Print and shaded views of the part. All mm, measured from the part's lowest x, y and z. Coordinates: 2 decimals unless noted, no trailing zeros. Loops run counter-clockwise (first coordinate to the right, second up) from the corner with the lowest first, then second, coordinate; pieces in that order, holes last. Notation, with made-up numbers: M 88.5,-6.5 L 111.5,-6.5 A24 cw 111.5,20.5 Z; hole C 87.25,-2.5 d8. An arc over 180 degrees is marked long. Use a Markdown table: item, result. Add a question column.
1) Pin check, flat tip, straight feed: pin 1 Ø1.1 at (x, z) = (1, 6.08) entering from -Y (3 decimals). Stop position of the tip, or through.
2) Band-saw the part on C-C (y = 0.7). State how many separate pieces and enclosed holes the cut face has, plus the area to 3 significant figures.
3) Band-saw the part on B-B (z = 8.62). List the corners of the cut face in (x, y) (3 decimals), plus the area to 3 significant figures.
4) Band-saw the part on D-D (x = 6). List the corners of the cut face in (y, z).
5) Wall check: probe 1 along Z at (x, y) = (1, 0.8) (3 decimals); probe 2 along Z at (x, y) = (5.75, 0.1). Give the ranges that are in metal, low to high. Write a range as from..to.
6) Band-saw the part on A-A (x = 13.7). List the corners of the cut face in (y, z) (3 decimals), plus the area to 3 significant figures.
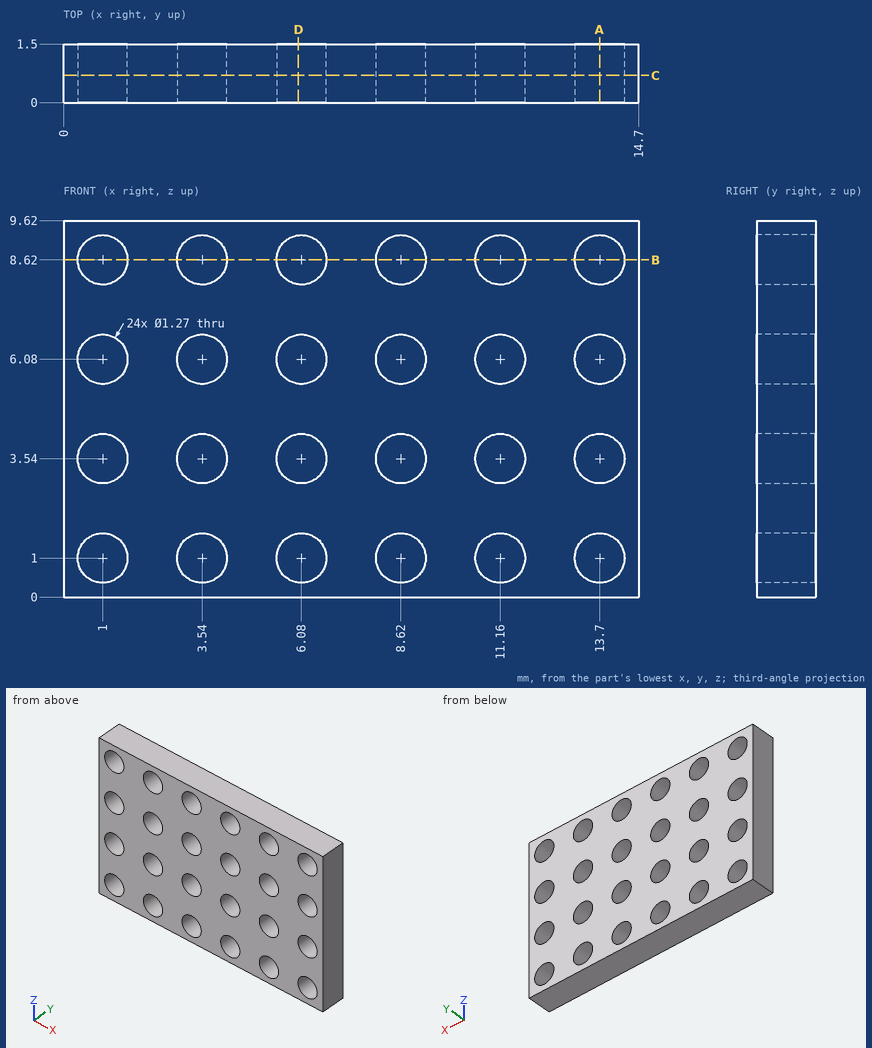
Entries:
| question | item | result |
|---|---|---|
| 1 | pin 1 | through |
| 2 | separate pieces | 1 |
| 2 | enclosed holes | 24 |
| 2 | area | 111 mm2 |
| 3 | outline | M 0,0 L 0.365,0 L 0.365,1.5 L 0,1.5 Z; M 1.635,0 L 2.905,0 L 2.905,1.5 L 1.635,1.5 Z; M 4.175,0 L 5.445,0 L 5.445,1.5 L 4.175,1.5 Z; M 6.715,0 L 7.985,0 L 7.985,1.5 L 6.715,1.5 Z; M 9.255,0 L 10.525,0 L 10.525,1.5 L 9.255,1.5 Z; M 11.795,0 L 13.065,0 L 13.065,1.5 L 11.795,1.5 Z; M 14.335,0 L 14.7,0 L 14.7,1.5 L 14.335,1.5 Z |
| 3 | area | 10.6 mm2 |
| 4 | outline | M 0,0 L 1.5,0 L 1.5,0.37 L 0,0.37 Z; M 0,1.63 L 1.5,1.63 L 1.5,2.91 L 0,2.91 Z; M 0,4.17 L 1.5,4.17 L 1.5,5.45 L 0,5.45 Z; M 0,6.71 L 1.5,6.71 L 1.5,7.99 L 0,7.99 Z; M 0,9.25 L 1.5,9.25 L 1.5,9.62 L 0,9.62 Z |
| 5 | probe 1 | 0..0.365, 1.635..2.905, 4.175..5.445, 6.715..7.985, 9.255..9.62 |
| 5 | probe 2 | 0..0.46, 1.54..3, 4.08..5.54, 6.62..8.08, 9.16..9.62 |
| 6 | outline | M 0,0 L 1.5,0 L 1.5,0.365 L 0,0.365 Z; M 0,1.635 L 1.5,1.635 L 1.5,2.905 L 0,2.905 Z; M 0,4.175 L 1.5,4.175 L 1.5,5.445 L 0,5.445 Z; M 0,6.715 L 1.5,6.715 L 1.5,7.985 L 0,7.985 Z; M 0,9.255 L 1.5,9.255 L 1.5,9.62 L 0,9.62 Z |
| 6 | area | 6.81 mm2 |
